Build history of the part. All positions in model axes, mm. Face numbers are marked on the shaded views. A direction names the side the tool comes from. Round coordinates to 2 decimals unless told otherwise and drop trailing zeros. Loops run counter-clockwise (first coordinate to the right, second up) from the corner with the lowest first, then second, coordinate; pieces in that order, holes last. Notation, with made-up numbers: M -27.75,32.25 L 18.25,32.25 A18 cw 18.25,60.25 Z; hole C 37.5,-18 d5. An arc over 180 degrees is marked long. One line per item, written item: value.
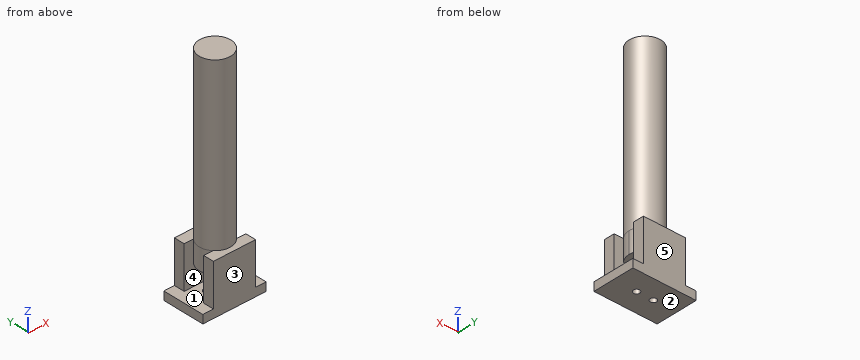
```python
from build123d import *

# Parameters (mm, degrees)
SKETCH_1_W           = 30
SKETCH_1_H           = 20
SKETCH_1_R           = 1.5
EXTRUDE_1_DEPTH      = 4
SKETCH_2_W           = 20
SKETCH_2_H           = 5
EXTRUDE_2_DEPTH      = 20
SKETCH_3_R           = 7.5
EXTRUDE_3_DEPTH      = 80
EXTRUDE_3_DEPTH_BACK = 10


with BuildPart() as part:
    # 草图1 → 凸台-拉伸1 (new body)
    with BuildSketch(Plane.XY):
        with Locations((1.097142857, 0.694285714)):
            Rectangle(SKETCH_1_W, SKETCH_1_H)
        with Locations((-2.902857143, 0.694285714)):
            Circle(SKETCH_1_R, mode=Mode.SUBTRACT)
        with Locations((5.097142857, 0.694285714)):
            Circle(SKETCH_1_R, mode=Mode.SUBTRACT)
    extrude(amount=EXTRUDE_1_DEPTH)

    # 草图2 → 凸台-拉伸2 (add)
    with BuildSketch(Plane.XY.offset(4)):
        with Locations((1.097142857, 8.194285714)):
            Rectangle(SKETCH_2_W, SKETCH_2_H)
        with Locations((1.097142857, -6.805714286)):
            Rectangle(SKETCH_2_W, SKETCH_2_H)
    extrude(amount=EXTRUDE_2_DEPTH)

    # 草图3 → 凸台-拉伸3 (add, two sides)
    with BuildSketch(Plane.XY.offset(24)) as extrude_3_sk:
        with Locations((1.097142857, 0.694285714)):
            Circle(SKETCH_3_R)
    extrude(amount=EXTRUDE_3_DEPTH)
    extrude(extrude_3_sk.sketch, amount=-EXTRUDE_3_DEPTH_BACK)


solid = part.part
```
Item 1: Slice it at C-C, the plane y = -2. Give the cut face in (x, z).
Check values:
outline: M -13.9,0 L 16.1,0 L 16.1,4 L -13.9,4 Z; M -5.9,14 L 8.1,14 L 8.1,104 L -5.9,104 Z
Item 2: Slice it at D-D, the plane z = 18. Give the cut face in (x, y), and give its area (3 significant figures).
Check values:
outline: M -8.9,-9.31 L 11.1,-9.31 L 11.1,-4.31 L 6.69,-4.31 A7.5 ccw 6.69,5.69 L 11.1,5.69 L 11.1,10.69 L -8.9,10.69 L -8.9,5.69 L -4.49,5.69 A7.5 ccw -4.49,-4.31 L -8.9,-4.31 Z
area: 338 mm2
Item 3: Slice it at B-B, the plane x = -7.5. Give the cut face in (y, z), and give its area (3 significant figures).
Check values:
outline: M -9.31,0 L 10.69,0 L 10.69,24 L 5.69,24 L 5.69,4 L -4.31,4 L -4.31,24 L -9.31,24 Z
area: 280 mm2
Item 4: Drop flat-ended pins along their axis: P1, Ø4, axis at x = 1, z = 62.5, coming from the +Y side; P2, Ø8, axis at y = 2, z = 29.5, coming from the +X side; P3, Ø12, axis at y = 7.5, z = 22.5, coming from the +X side. Give the stop position or say it passes through.
Check values:
P1: stops at y = 8.19
P2: stops at x = 8.6
P3: stops at x = 11.1
Item 5: Slice it at A-A, the plane z = 7.5. Give the cut face in (x, y), and give its area (3 significant figures).
Check values:
outline: M -8.9,-9.31 L 11.1,-9.31 L 11.1,-4.31 L -8.9,-4.31 Z; M -8.9,5.69 L 11.1,5.69 L 11.1,10.69 L -8.9,10.69 Z
area: 200 mm2
Item 6: Which spindle directions (+Z, -Z, +X, -X, +Y, -Y) get a long thin tool onto all of the face, cutting with end or side? Do the marked faces 4 and 5. Say none if no direction does.
Check values:
face 4: none
face 5: +Z, -Z, +X, -X, +Y
Item 7: Wall check: line 1 along Z through (x, y) = (-1.75, -1); line 2 along Y through (x, z) = (-1.5, 9.5); line 3 along X through (y, z) = (1, 63). Give the ranges that are in metal, low to high.
Check values:
line 1: z = 0 to 4, 14 to 104
line 2: y = -9.31 to -4.31, 5.69 to 10.69
line 3: x = -6.4 to 8.59
Item 8: Pull direction Z, two halves, no side cores. Call the marked faces 1, 2 and 3: pulls with the +Z half, pulls with the -Z half, needs draft (parallel to the pull), parting line crosses it, or undercut.
Check values:
face 1: undercut
face 2: pulls with the -Z half
face 3: needs draft
